Source: CAD feature listing. Evaluate the final solid. Frame: model axes, mm. A direction names the side the tool comes from. Give positions to 0.01 mm unless a question says otherwise; leave off trailing zeros. Loops run counter-clockwise (first coordinate to the right, second up) from the corner with the lowest first, then second, coordinate; pieces in that order, holes last. Notation, with made-up numbers: M 52.5,47 L 99.5,47 A17 cw 99.5,58 Z; hole C -6.75,-34.5 d6. An arc over 180 degrees is marked long. Put each result on its own line as item: value.
from build123d import *

# Parameters (mm, degrees)
F0_R      = 7
F1_DEPTH  = 25
F3_DEPTH  = 10
F4_R      = 10.5
F5_DEPTH  = 14
F7_DEPTH  = 55
F8_R      = 7.49999
F10_DEPTH = 20
F12_DEPTH = 33
F13_SIZE2 = 5
F13_SIZE  = 5
F15_DEPTH = 400


# Not quite as in the source:
# - a fillet or chamfer is up to 0.001 mm smaller than in the source, because OpenCascade refuses the exact size


with BuildPart() as f1:
    # F0 (on Front) → F1 (new body)
    with BuildSketch(Plane.XZ):
        with BuildLine():
            ThreePointArc((-183, -20), (-180.0710678119, -27.0710678119), (-173, -30))
            Line((-173, -30), (20, -30))
            ThreePointArc((20, -30), (27.0710678119, -27.0710678119), (30, -20))
            Line((30, -20), (30, 160))
            ThreePointArc((30, 160), (27.0710678119, 167.0710678119), (20, 170))
            Line((20, 170), (-173, 170))
            ThreePointArc((-173, 170), (-180.0710678119, 167.0710678119), (-183, 160))
            Line((-183, 160), (-183, -20))
        make_face()
        Circle(F0_R, mode=Mode.SUBTRACT)
    extrude(amount=F1_DEPTH)

    # F2 (on face) → F3 (join)
    with BuildSketch(Plane.XZ.offset(25)):
        with BuildLine():
            Line((-30, 15), (-30, -30))
            Line((-30, -30), (20, -30))
            ThreePointArc((20, -30), (27.0710678119, -27.0710678119), (30, -20))
            Line((30, -20), (30, 30))
            Line((30, 30), (-15, 30))
            ThreePointArc((-15, 30), (-25.6066017178, 25.6066017178), (-30, 15))
        make_face()
    extrude(amount=F3_DEPTH)

    # F4 (on face) → F5 (cut)
    with BuildSketch(Plane.XZ.offset(35)):
        Circle(F4_R)
    extrude(amount=-F5_DEPTH, mode=Mode.SUBTRACT)

    # F6 (on face) → F7 (join)
    with BuildSketch(Plane.XZ.offset(25)):
        with BuildLine():
            Line((-140, 30), (-140, -30))
            Line((-140, -30), (-125, -30))
            Line((-125, -30), (-125, 30))
            ThreePointArc((-125, 30), (-122.8526407389, 36.191609922), (-117.3327933147, 39.7240976625))
            ThreePointArc((-117.3327933147, 39.7240976625), (-67.5809110947, 67.5809110947), (-39.7240976625, 117.3327933147))
            ThreePointArc((-39.7240976625, 117.3327933147), (-36.191609922, 122.8526407389), (-30, 125))
            Line((-30, 125), (30, 125))
            Line((30, 125), (30, 140))
            Line((30, 140), (-30, 140))
            ThreePointArc((-30, 140), (-45.479024805, 134.6316018472), (-54.3102441564, 120.8319832868))
            ThreePointArc((-54.3102441564, 120.8319832868), (-78.1875128125, 78.1875128125), (-120.8319832868, 54.3102441564))
            ThreePointArc((-120.8319832868, 54.3102441564), (-134.6316018472, 45.479024805), (-140, 30))
        make_face()
    extrude(amount=F7_DEPTH)

    # F8 (radius 7.5 in the source; OpenCascade refuses exactly that, so slightly less here)
    f8_edges = [f1.edges().sort_by_distance(p)[0] for p in [
        (-125, -80, 0),
        (-140, -80, 0),
    ]]
    fillet(f8_edges, radius=F8_R)

    # F9 (on face) → F10 (cut)
    with BuildSketch(Plane.XZ.offset(25)):
        with BuildLine():
            ThreePointArc((-108.8892841225, 32.6891427357), (-114.0278528021, 29.0783179154), (-116, 23.1156356845))
            Line((-116, 23.1156356845), (-116, -11))
            ThreePointArc((-116, -11), (-113.0710678119, -18.0710678119), (-106, -21))
            Line((-106, -21), (-49, -21))
            ThreePointArc((-49, -21), (-41.9289321881, -18.0710678119), (-39, -11))
            Line((-39, -11), (-39, 15))
            ThreePointArc((-39, 15), (-31.9705627485, 31.9705627485), (-15, 39))
            Line((-15, 39), (21, 39))
            Line((21, 39), (21, 106))
            ThreePointArc((21, 106), (18.0710678119, 113.0710678119), (11, 116))
            Line((11, 116), (-23.1156356845, 116))
            ThreePointArc((-23.1156356845, 116), (-29.0783179154, 114.0278528021), (-32.6891427357, 108.8892841225))
            ThreePointArc((-32.6891427357, 108.8892841225), (-61.216950064, 61.216950064), (-108.8892841225, 32.6891427357))
        make_face()
    extrude(amount=-F10_DEPTH, mode=Mode.SUBTRACT)

    # F11 (on face) → F12 (join)
    with BuildSketch(Plane.XZ.offset(25)):
        with BuildLine():
            Line((-70.8271231193, 161), (-164, 161))
            ThreePointArc((-164, 161), (-171.0710678119, 158.0710678119), (-174, 151))
            Line((-174, 151), (-174, 70.8271231193))
            ThreePointArc((-174, 70.8271231193), (-171.0710678119, 63.7560553074), (-164, 60.8271231193))
            Line((-164, 60.8271231193), (-141.8271231193, 60.8271231193))
            ThreePointArc((-141.8271231193, 60.8271231193), (-84.5514738432, 84.5514738432), (-60.8271231193, 141.8271231193))
            Line((-60.8271231193, 141.8271231193), (-60.8271231193, 151))
            ThreePointArc((-60.8271231193, 151), (-63.7560553074, 158.0710678119), (-70.8271231193, 161))
        make_face()
    extrude(amount=F12_DEPTH)

    # F13
    f13_edges = [f1.edges().sort_by_distance(p)[0] for p in [
        (-174, -58, 110.913562),
    ]]
    chamfer(f13_edges, length=F13_SIZE, length2=F13_SIZE2)

    # F14 (on face) → F15 (cut)
    with BuildSketch(Plane(origin=(0, 0, -30), x_dir=(1, 0, 0), z_dir=(0, 0, -1))):
        with BuildLine():
            Line((-12.6804448871, 0), (12.6804448871, 0))
            ThreePointArc((12.6804448871, 0), (0, 12.6804448871), (-12.6804448871, 0))
        make_face()
    extrude(amount=-F15_DEPTH, mode=Mode.SUBTRACT)


solid = f1.part
1. Section query D-D (x = 0). State how many separate pieces and enclosed holes the cut face has, plus the area to 3 significant figures.
Found:
separate pieces: 3
enclosed holes: 0
area: 2,510 mm^2
2. Section query A-A (y = -43). Output: boundary loops of the cut face in (x, z).
Found:
outline: M -174,70.83 A10 ccw -164,60.83 L -141.83,60.83 A81 ccw -60.83,141.83 L -60.83,151 A10 ccw -70.83,161 L -164,161 A10 ccw -174,151 Z; M -140,-30 L -125,-30 L -125,30 A10 cw -117.33,39.72 A105 ccw -39.72,117.33 A10 cw -30,125 L 30,125 L 30,140 L -30,140 A25 ccw -54.31,120.83 A90 cw -120.83,54.31 A25 ccw -140,30 Z
3. Access query for faces 5 (the flat face through (-117, -39, 161)), 6 (the cylindrical face through (-42.01, -15.14, -18.15)), 7 (the flat face through (-125, -48, 0)), 8 (the cylindrical face through (-63.679, -38.804, 157.993)). Directions: +Z, -Z, +X, -X, +Y, -Y. A direction counts if a zero-diameter tool reaches every point of the face in a straight line with its end or side. Return the directions, or none.
Found:
face 5: +Z, +X, -X, -Y
face 6: -Y
face 7: -Z, -Y
face 8: +Z, +X, -Y
4. Section query C-C (y = -31.5). Output: boundary loops of the cut face in (x, z), plus the area to 3 significant figures.
Found:
outline: M -174,70.83 A10 ccw -164,60.83 L -141.83,60.83 A81 ccw -60.83,141.83 L -60.83,151 A10 ccw -70.83,161 L -164,161 A10 ccw -174,151 Z; M -140,-30 L -125,-30 L -125,30 A10 cw -117.33,39.72 A105 ccw -39.72,117.33 A10 cw -30,125 L 30,125 L 30,140 L -30,140 A25 ccw -54.31,120.83 A90 cw -120.83,54.31 A25 ccw -140,30 Z; M -30,-30 L 20,-30 A10 ccw 30,-20 L 30,30 L -15,30 A15 ccw -30,15 Z; hole C 0,0 d21
area: 17,200 mm^2
5. Draft query along Z for faces 1 (the cylindrical face through (-171.148, -38.804, 63.834)), 2 (the conical face through (-88.51, -57.76, 87.33)), 3 (the cylindrical face through (-137.861, -77.745, -0.42)), 4 (the flat face through (-116, -15, 6)). Return one class per face: pulls with the +Z half, pulls with the -Z half, needs draft (parallel to the pull), parting line crosses it, or undercut.
Found:
face 1: pulls with the -Z half
face 2: undercut
face 3: needs draft
face 4: undercut
6. Material intervals for line 1 (Z direction, x = 0, y = -16); line 2 (Z direction, x = 0, y = -31); line 3 (Y direction, x = -129.5, z = 104), sorted ascending. Write a range as from..to.
Found:
line 1: -30..-7, 7..39, 116..170
line 2: -30..-10.5, 10.5..30, 125..140
line 3: -58..0
7. Contact query for flat-ended pins moving along their axis: P1, Ø8, axis at x = -99.5, z = 135.5, coming from the -Y side; P2, Ø1.5, axis at y = -30, z = 20, coming from the -X side; P3, Ø8, axis at x = -14, z = 6, coming from the -Y side. Output: stop coordinate, or through.
Found:
P1: y = -58
P2: x = -140
P3: y = -35
